Geometry check sheet. Reference: the model listing, model coordinates, mm. Face numbers are marked on the shaded views. A direction names the side the tool comes from. Give positions to 0.01 mm unless a question says otherwise; leave off trailing zeros. Write each loop counter-clockwise with the first axis right and the second up, starting at its lowest first coordinate (ties: lowest second). Pieces come first, ordered by that corner, then holes. Notation, with made-up numbers: (-21.5, 36) -> (6.5, 36) arc R19 cw to (6.5, 41) -> close; hole circle Ø4 at (42.25, 24.25). An arc over 180 degrees is marked (long way). Use a Markdown table: item, result. Add a question column.
from build123d import *

# Parameters (mm, degrees)
F0_W     = 32
F0_H     = 40
F1_DEPTH = 2.5
F2_W     = 32
F2_H     = 20
F3_DEPTH = 7.5
F4_R     = 1.6
F5_DEPTH = 2.501
F6_R     = 2.6
F7_DEPTH = 20


with BuildPart() as f1:
    # F0 (on Front) → F1 (new body)
    with BuildSketch(Plane.XZ):
        with Locations((-16.529805, -15.329495)):
            Rectangle(F0_W, F0_H)
    extrude(amount=F1_DEPTH)

    # F2 (on face) → F3 (join)
    with BuildSketch(Plane.XZ.offset(2.5)):
        with Locations((-16.529805, -5.329495)):
            Rectangle(F2_W, F2_H)
    extrude(amount=F3_DEPTH)

    # F4 (on face) → F5 (cut, through all)
    with BuildSketch(Plane.XZ.offset(2.5)):
        with Locations((-25.029805, -32.829495)):
            Circle(F4_R)
        with BuildLine():
            ThreePointArc((-6.37738, -32.856394), (-6.377437, -32.842944), (-6.377607, -32.829495))
            ThreePointArc((-6.377607, -32.829495), (-9.577324, -32.869844), (-6.37738, -32.856394))
        make_face()
    extrude(amount=-F5_DEPTH, mode=Mode.SUBTRACT)

    # F6 (on face) → F7 (cut, through all)
    with BuildSketch(Plane.XY.offset(4.670505)):
        with Locations((-16.529805, -10)):
            Circle(F6_R)
    extrude(amount=-F7_DEPTH, mode=Mode.SUBTRACT)


solid = f1.part
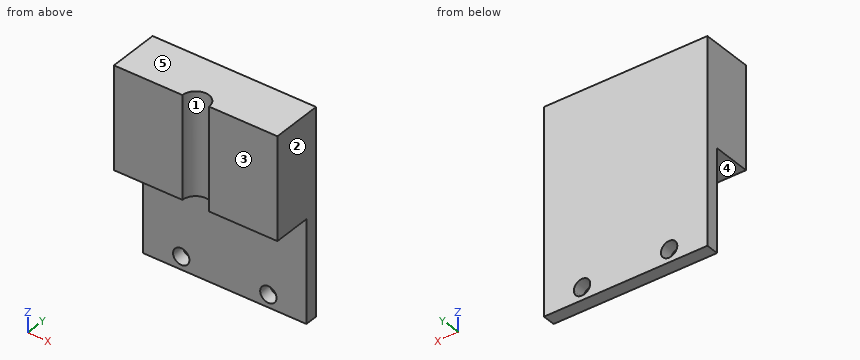
1) Material ranges on probe 1 along Z at (x, y) = (-4.5, -9.25); probe 2 along Y at (x, z) = (-16.5, -14.5); probe 3 along Y at (x, z) = (-11, -33), recorded low to high. Write a range as [from, to].
2) Sectioned sample at B-B, the plane z = -10. Enter the section's corners in (x, y), and give its area (3 significant figures).
3) Gauge pin test, flat ends, axial feed: P1, Ø10, axis at x = -13, z = -30, coming from the -Y side; P2, Ø6, axis at x = -16, y = -7, coming from the -Z side. Record the tip position at first contact, or that the pin passes through.
4) Sectioned sample at D-D, the plane x = -4.5. Enter the section's corners in (y, z), and give its area (3 significant figures).
5) Sectioned sample at A-A, the plane y = -9.5. Enter the section's corners in (x, z).
6) Draft check along X on the marked faces 1, 2 and 3. Enter one of: +X half, -X half, draft (parallel to the pull), parting line (faces both ways), or undercut.
7) Sectioned sample at C-C, the plane x = -25. Enter the section's corners in (y, z), and give its area (3 significant figures).
8) Tool access check on the marked faces 4 and 5. Record the directions out of +Z, -Z, +X, -X, +Y, -Y that give a thin tool (end or side, any length) a straight path to the whole face; none if there is none.
Check values:
| question | item | result |
|---|---|---|
| 1 | probe 1 | [-15.33, 4.67] |
| 1 | probe 2 | [-7.4, 0] |
| 1 | probe 3 | [-2.5, 0] |
| 2 | outline | (-32.53, -10) -> (-19.13, -10) arc R2.6 cw to (-13.93, -10) -> (-0.53, -10) -> (-0.53, 0) -> (-32.53, 0) -> close |
| 2 | area | 309 mm² |
| 3 | P1 | y = -2.5 |
| 3 | P2 | z = -15.33 |
| 4 | outline | (-10, -15.33) -> (-2.5, -15.33) -> (-2.5, -35.33) -> (0, -35.33) -> (0, 4.67) -> (-10, 4.67) -> close |
| 4 | area | 250 mm² |
| 5 | outline | (-32.53, -15.33) -> (-19.08, -15.33) -> (-19.08, 4.67) -> (-32.53, 4.67) -> close; (-13.98, -15.33) -> (-0.53, -15.33) -> (-0.53, 4.67) -> (-13.98, 4.67) -> close |
| 6 | face 1 | undercut |
| 6 | face 2 | +X half |
| 6 | face 3 | draft |
| 7 | outline | (-10, -15.33) -> (-2.5, -15.33) -> (-2.5, -31.23) -> (0, -31.23) -> (0, 4.67) -> (-10, 4.67) -> close; (-2.5, -35.33) -> (0, -35.33) -> (0, -34.43) -> (-2.5, -34.43) -> close |
| 7 | area | 242 mm² |
| 8 | face 4 | -Z, +X, -X, -Y |
| 8 | face 5 | +Z, +X, -X, +Y, -Y |
